```python
from build123d import *

# Parameters (mm, degrees)
F0_W     = 2.8
F0_H     = 9
F1_DEPTH = 19.8
F3_F1_R  = 5
F3_F2_R  = 5
F4_DEPTH = 6
F5_R     = 5


# Not quite as in the source:
# - a feature of the source that left no trace in its solid (it failed there, or was rolled back) is left out


with BuildPart() as f1:
    # F0 (on Right) → F1 (new body)
    with BuildSketch(Plane.YZ):
        Polygon((0, 9), (0, 0), (3, 0), (3, 2.7590821834), (3, 9), align=None)
        with Locations((8.6, 4.5)):
            Rectangle(F0_W, F0_H)
        Polygon((3, 0), (0, 0), (0, -3), (7.832443736, -3), (5.3151448425, 0), align=None)
        Polygon((7.2, 0), (5.3151448425, 0), (7.832443736, -3), (10, -3), (10, 0), align=None)
        Polygon((0, -3), (0, 0), (-6, 0), (-6, -40), (20.0199263242, -30.5295213202), (11.6604444312, -7.562033581), (7.832443736, -3), align=None)
        Polygon((10, -3), (7.832443736, -3), (11.6604444312, -7.562033581), align=None)
        Polygon((28.3794082171, -27.4869187373), (11.6604444312, -7.562033581), (20.0199263242, -30.5295213202), align=None)
    extrude(amount=F1_DEPTH)

    # F3: fillet of radius 5 on 6 edges, made by hand

    # F3_f1
    f3_f1_edges = [f1.edges().sort_by_distance(p)[0] for p in [
        (9.9, 10, -3),
        (9.9, 11.6604444312, -7.562033581),
    ]]
    fillet(f3_f1_edges, radius=F3_F1_R)

    # F3_f2
    f3_f2_edges = [f1.edges().sort_by_distance(p)[0] for p in [
        (0, -6, -20),
        (19.8, -6, -20),
        (19.8, 20.3032783203, -17.8621619185),
        (0, 20.3032783203, -17.8621619185),
        (0, 11.7272436201, -7.5234670512),
        (19.8, 11.7272436201, -7.5234670512),
    ]]
    fillet(f3_f2_edges, radius=F3_F2_R)

    # F2 (on face) → F4 (cut, through all)
    with BuildSketch(Plane.XZ.offset(6)):
        with BuildLine():
            ThreePointArc((4.9, 0), (9.9, -2), (14.9, 0))
            Line((14.9, 0), (4.9, 0))
        make_face()
    extrude(amount=-F4_DEPTH, mode=Mode.SUBTRACT)

    # F5
    f5_edges = [f1.edges().sort_by_distance(p)[0] for p in [
        (14.9, -2.9995, 0),
        (4.9, -2.9995, 0),
    ]]
    fillet(f5_edges, radius=F5_R)


solid = f1.part
```
Geometry check sheet. Reference: the model listing, model coordinates, mm. A direction names the side the tool comes from. Round coordinates to 2 decimals unless told otherwise and drop trailing zeros. Loops run counter-clockwise (first coordinate to the right, second up) from the corner with the lowest first, then second, coordinate; pieces in that order, holes last. Notation, with made-up numbers: (2, 27) -> (27, 27) arc R21 ccw to (27, 57) -> close; hole circle Ø10 at (50.5, 74.25). An arc over 180 degrees is marked (long way). Use a Markdown table: item, result.
(1) Scan lines: probe 1 along Y at (x, z) = (8.75, 5); probe 2 along Y at (x, z) = (18.75, -13); probe 3 along X at (y, z) = (-1.5, -15). Record each from-to range of solid material in increasing order.
Calculated:
| item | result |
|---|---|
| probe 1 | 0 to 3, 7.2 to 10 |
| probe 2 | -4.07 to 13.7 |
| probe 3 | 0.03 to 19.77 |
(2) Sectioned sample at A-A (x = 9.5). Enter the section's corners in (y, z).
Calculated:
| item | result |
|---|---|
| outline | (-6, -40) -> (28.38, -27.49) -> (12.23, -8.24) arc R5 cw to (11.36, -6.73) -> (10.3, -3.83) arc R5 cw to (10, -2.12) -> (10, 9) -> (7.2, 9) -> (7.2, 0) -> (3, 0) -> (3, 9) -> (0, 9) -> (0, -1.99) -> (-6, -1.99) -> close |
(3) Go/stop test with flat-tipped pins: P1, Ø2.5, axis at x = 18.5, y = -4, coming from the +Z side; P2, Ø5, axis at x = 10, z = 3, coming from the +Y side; P3, Ø8, axis at x = 7, z = -3.5, coming from the +Y side; P4, Ø10, axis at x = 4.5, z = -14, coming from the -Y side. Record where each tip stops, or that it passes through.
Calculated:
| item | result |
|---|---|
| P1 | z = 0 |
| P2 | y = 10 |
| P3 | y = 11.71 |
| P4 | y = -6 |
(4) Set-up check for faces 4 (the flat face through (2, -2, 0)), 5 (the cylindrical face through (4.601, -2.958, -0.203)), 6 (the cylindrical face through (2, 9, 4)), 7 (the flat face through (10, 5, 0)): record each of +Z, -Z, +X, -X, +Y, -Y from which the full face is reachable in a straight line by a thin tool's end or side.
Calculated:
| item | result |
|---|---|
| face 4 | +Z, +X, -X, -Y |
| face 5 | +Z, -Y |
| face 6 | +Z, -X, +Y |
| face 7 | +Z, +X, -X |
(5) Sectioned sample at B-B (y = -2). Enter the section's corners in (x, z).
Calculated:
| item | result |
|---|---|
| outline | (0.1, -38.54) -> (19.7, -38.54) -> (19.7, 0) -> (16.61, 0) arc R5 ccw to (13.87, -0.82) arc R7.25 cw to (5.93, -0.82) arc R5 ccw to (3.19, 0) -> (0.1, 0) -> close |
(6) Sectioned sample at C-C (x = 2.5). Enter the section's corners in (y, z).
Calculated:
| item | result |
|---|---|
| outline | (-5.33, -39.76) -> (27.71, -27.73) -> (11.71, -8.67) arc R5.67 cw to (10.73, -6.96) -> (9.67, -4.06) arc R5.67 cw to (9.33, -2.12) -> (9.33, 9) -> (7.2, 9) -> (7.2, 0) -> (3, 0) -> (3, 9) -> (0, 9) -> (0, 0) -> (-5.33, 0) -> close |
(7) Mould release check, pull along Y, two halves, no side actions. Record for faces 1 (the flat face through (0, 6, -20)), 2 (the flat face through (10, -6, -20)), 3 (the flat face through (10, 7.2, 4)): released by +Y, released by -Y, zero draft, split by the parting line, or undercut.
Calculated:
| item | result |
|---|---|
| face 1 | zero draft |
| face 2 | released by -Y |
| face 3 | undercut |
